Autodesk Inventor part; units mm, degrees
ref_plane "YZ Plane" through (0, 0, 0) normal (1, 0, 0) x (0, 1, 0)
ref_plane "XZ Plane" through (0, 0, 0) normal (0, 1, 0) x (-1, 0, 0)
ref_plane "XY Plane" through (0, 0, 0) normal (0, 0, 1) x (1, 0, 0)
sketch "Skizze1" plane through (0, 0, 0) normal (0, 1, 0) x (-1, 0, 0)
  circle A0 centre (0, 0) radius 8
  dimension "d0" = 16
extrude "Extrusion1" add sketch "Skizze1" along normal blind 6.5
sketch "Skizze2" plane through (0, 0, 0) normal (0, -1, 0) x (1, 0, 0)
  circle A0 centre (0, 0) radius 5
  dimension "d3" = 10
extrude "Extrusion2" add sketch "Skizze2" along normal blind 4.5
sketch "Skizze3" plane through (0, -4.5, 0) normal (0, -1, 0) x (1, 0, 0)
  circle A0 centre (0, 0) radius 5
hole "Bohrung1" at (0, -4.5, 0) direction (0, 1, 0) diameter 7 depth 5.5 tip angle 118
sketch "Skizze4" plane through (0, 6.5, 0) normal (0, 1, 0) x (1, 0, 0)
  circle A0 centre (0, 0) radius 8
hole "Bohrung2" at (0, 6.5, 0) direction (0, -1, 0) diameter 12 depth 5
chamfer "Fasen1" distance 0.6 angle 45 2 edges at (8, 6.5, 0) (8, 0, 0)
properties part number "8"
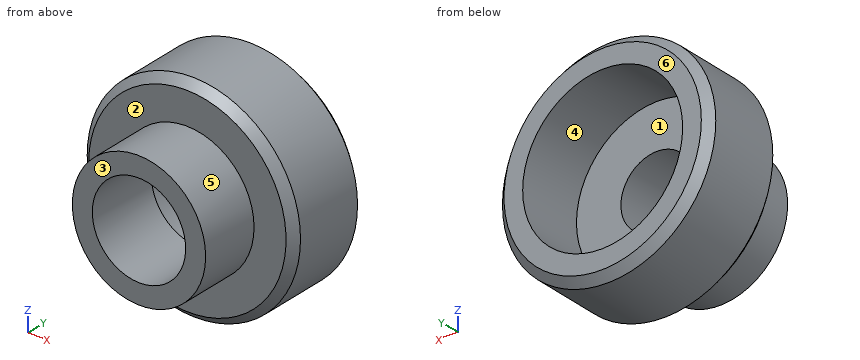
For this review, take the finished solid that the model builds, in its own axes (mm). Face numbers are marked on the shaded views. A direction names the side the tool comes from. Round coordinates to 2 decimals unless told otherwise and drop trailing zeros. Order: outer loops, then holes, each group sorted by start corner. A loop starts at its lowest first (then second) coordinate and runs counter-clockwise, first axis right, second up. Notation, with made-up numbers: (54, 86.5) -> (80, 86.5) arc R23 cw to (80, 125.5) -> close; hole circle Ø1 at (28, 25). An arc over 180 degrees is marked (long way). Put each result on its own line as item: value.
Q1. Mouldability with a two-part tool opening along Z and no side actions: class the marked faces 4, 5 and 6 as pulls with the +Z half, pulls with the -Z half, needs draft (parallel to the pull), parting line crosses it, or undercut.
Check result:
face 4: undercut
face 5: parting line crosses it
face 6: needs draft
Q2. Add section A-A on x = 0. Write out the cut boundary in (y, z).
Check result:
outline: (-4.5, -5) -> (0, -5) -> (0, -7.4) -> (0.6, -8) -> (5.9, -8) -> (6.5, -7.4) -> (6.5, -6) -> (1.5, -6) -> (1.5, -2.67) -> (1, -3.5) -> (-4.5, -3.5) -> close; (-4.5, 3.5) -> (1, 3.5) -> (1.5, 2.67) -> (1.5, 6) -> (6.5, 6) -> (6.5, 7.4) -> (5.9, 8) -> (0.6, 8) -> (0, 7.4) -> (0, 5) -> (-4.5, 5) -> close
Q3. Add section C-C on z = 0. Write out the cut boundary in (x, y), plus the area to 3 significant figures.
Check result:
outline: (-8, 0.6) -> (-7.4, 0) -> (-5, 0) -> (-5, -4.5) -> (-3.5, -4.5) -> (-3.5, 1) -> (-2.67, 1.5) -> (-6, 1.5) -> (-6, 6.5) -> (-7.4, 6.5) -> (-8, 5.9) -> close; (2.67, 1.5) -> (3.5, 1) -> (3.5, -4.5) -> (5, -4.5) -> (5, 0) -> (7.4, 0) -> (8, 0.6) -> (8, 5.9) -> (7.4, 6.5) -> (6, 6.5) -> (6, 1.5) -> close
area: 46.7 mm2
Q4. Insertion check: pin 1 Ø5 at (y, z) = (3.5, 2.5) entering from -X; pin 2 Ø4 at (y, z) = (2, 4) entering from +X; pin 3 Ø9 at (x, z) = (0, 0) entering from +Y; pin 4 Ø3 at (x, y) = (2.5, -2) entering from -Z. Each pin has a flat end and moves straight along its axis. Give the tip position at first contact, or say it passes through.
Check result:
pin 1: x = -8
pin 2: x = 7.75
pin 3: y = 1.5
pin 4: z = -4.9
Q5. Add section B-B on y = -2.5. Write out the cut boundary in (x, z).
Check result:
outline: circle Ø10 at (0, 0); hole circle Ø7 at (0, 0)
Q6. For probe 1 along Z at (x, y) = (0, -1.2); probe 2 along Z at (x, y) = (0, 4.65); probe 3 along Y at (x, z) = (1.5, 3.75), list the stretches that pass through material, from the lowest coordinate up. Write a range as [from, to].
Check result:
probe 1: [-5, -3.5], [3.5, 5]
probe 2: [-8, -6], [6, 8]
probe 3: [-4.5, 1.5]
Q7. Machinability: for the marked faces 1, 2 and 3, which of the approach directions +Z, -Z, +X, -X, +Y, -Y give a long, thin tool a straight path to every point of the face, cutting with its end or side? Answer none if there is none.
Check result:
face 1: +Y
face 2: -Y
face 3: +Z, -Z, +X, -X, -Y
Q8. Add section D-D on y = 4.25. Write out the cut boundary in (x, z), plus the area to 3 significant figures.
Check result:
outline: circle Ø16 at (0, 0); hole circle Ø12 at (0, 0)
area: 88.0 mm2
